```python
from build123d import *

# Parameters (mm, degrees)
SKETCH_1_W         = 140
SKETCH_1_H         = 95
EXTRUDE_1_DEPTH    = 10
HOLE_WIZARD_M4_1_D = 3.3
HOLE_WIZARD_M6_1_D = 5


with BuildPart() as part:
    # 草图1 → 凸台-拉伸1 (new body)
    with BuildSketch(Plane.XY):
        with Locations((70, 47.5)):
            Rectangle(SKETCH_1_W, SKETCH_1_H)
    extrude(amount=EXTRUDE_1_DEPTH)

    # M4 螺纹孔1 (through all)
    with Locations(Plane(origin=(4.65, 83.45, 10), x_dir=(1, 0, 0), z_dir=(0, 0, 1))):
        with Locations((0, 0), (0, -26), (26, -26), (26, 0), (104.7, 0), (130.7, 0), (130.7, -26), (104.7, -26), (39.5, -59.45), (39.5, -77.45), (91.2, -59.45), (91.2, -77.45)):
            Hole(HOLE_WIZARD_M4_1_D / 2)

    # M6 螺纹孔1 (through all)
    with Locations(Plane(origin=(30, 32, 10), x_dir=(1, 0, 0), z_dir=(0, 0, 1))):
        with Locations((0, 0), (0, -24), (80, 0), (80, -24)):
            Hole(HOLE_WIZARD_M6_1_D / 2)


solid = part.part
```
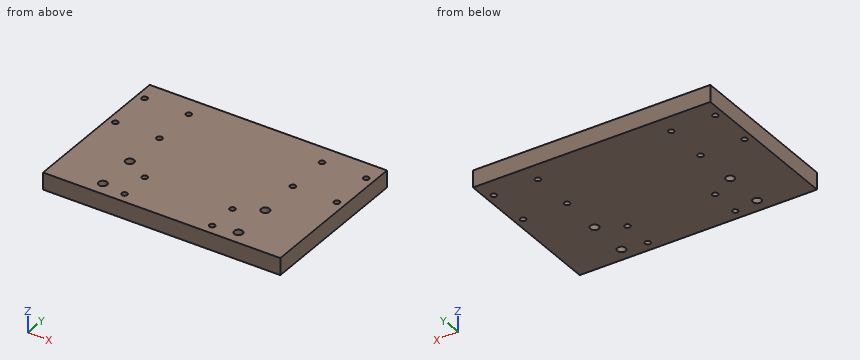
Geometry: final body of the model. Coordinates: model frame, mm. Round coordinates to 2 decimals unless told otherwise and drop trailing zeros. Order: outer loops, then holes, each group sorted by start corner. A loop starts at its lowest first (then second) coordinate and runs counter-clockwise, first axis right, second up. Notation, with made-up numbers: M 55.5,63 L 95.5,63 A24 cw 95.5,77 Z; hole C 80.25,56 d3. An arc over 180 degrees is marked long. One line per item, written item: value.
(1) Cut plane C-C (y = 57.45). Return the cut outline in (x, z).
Result sheet:
outline: M 0,0 L 3,0 L 3,10 L 0,10 Z; M 6.3,0 L 29,0 L 29,10 L 6.3,10 Z; M 32.3,0 L 107.7,0 L 107.7,10 L 32.3,10 Z; M 111,0 L 133.7,0 L 133.7,10 L 111,10 Z; M 137,0 L 140,0 L 140,10 L 137,10 Z
(2) Cut plane D-D (x = 109.35). Return the cut outline in (y, z), and give its area (3 significant figures).
Result sheet:
outline: M 0,0 L 5.59,0 L 5.59,10 L 0,10 Z; M 10.41,0 L 29.59,0 L 29.59,10 L 10.41,10 Z; M 34.41,0 L 55.8,0 L 55.8,10 L 34.41,10 Z; M 59.1,0 L 81.8,0 L 81.8,10 L 59.1,10 Z; M 85.1,0 L 95,0 L 95,10 L 85.1,10 Z
area: 787 mm2
(3) Line query: probe 1 along X at (y, z) = (83.45, 6); probe 2 along Y at (x, z) = (95.85, 5.5); probe 3 along X at (y, z) = (84, 9.5). Output: solid intervals per line, ascending. Write a range as [from, to].
Result sheet:
probe 1: [0, 3], [6.3, 29], [32.3, 107.7], [111, 133.7], [137, 140]
probe 2: [0, 4.35], [7.65, 22.35], [25.65, 95]
probe 3: [0, 3.09], [6.21, 29.09], [32.21, 107.79], [110.91, 133.79], [136.91, 140]
(4) Cut plane B-B (x = 44.15). Return the cut outline in (y, z), and give its area (3 significant figures).
Result sheet:
outline: M 0,0 L 4.35,0 L 4.35,10 L 0,10 Z; M 7.65,0 L 22.35,0 L 22.35,10 L 7.65,10 Z; M 25.65,0 L 95,0 L 95,10 L 25.65,10 Z
area: 884 mm2
(5) Cut plane A-A (y = 32). Return the cut outline in (x, z), and give its area (3 significant figures).
Result sheet:
outline: M 0,0 L 27.5,0 L 27.5,10 L 0,10 Z; M 32.5,0 L 107.5,0 L 107.5,10 L 32.5,10 Z; M 112.5,0 L 140,0 L 140,10 L 112.5,10 Z
area: 1,300 mm2
